```python
from build123d import *

# Parameters (mm, degrees)
F0_R     = 35
F1_DEPTH = 30
F4_DEPTH = 25
F6_D     = 60


with BuildPart() as f1:
    # F0 (on Top) → F1 (new body)
    with BuildSketch(Plane.XY):
        Circle(F0_R)
    extrude(amount=F1_DEPTH)

    # F3 (on offset) → F4 (join)
    with BuildSketch(Plane.YZ.offset(10)):
        Polygon((31.227464, 30), (31.227464, 0), (60.99254, 48.721532), (210.99254, 48.721532), (210.99254, 56.721532), (60.99254, 56.721532), align=None)
    extrude(amount=-F4_DEPTH)

    # F6 (through all)
    with Locations(Plane.XY.offset(30)):
        with Locations((0, 0)):
            Hole(F6_D / 2)


solid = f1.part
```
Verification items for the finished model (mm, model axes). A direction names the side the tool comes from. Give positions to 0.01 mm unless a question says otherwise; leave off trailing zeros. Write each loop counter-clockwise with the first axis right and the second up, starting at its lowest first coordinate (ties: lowest second). Pieces come first, ordered by that corner, then holes. Notation, with made-up numbers: (57, 16.25) - (111, 16.25) arc R30 cw to (111, 52.25) - close; hole circle Ø4 at (-14, 45.5). An arc over 180 degrees is marked (long way). Put each result on its own line as item: value.
Q1. Scan lines: probe 1 along X at (y, z) = (-24, 29); probe 2 along Y at (x, z) = (13.5, 23.5); probe 3 along Y at (x, z) = (-19, 27). Record each from-to range of solid material in increasing order. Write a range as from..to.
Result:
probe 1: -25.48..-18, 18..25.48
probe 2: -32.29..-26.79, 26.79..32.29
probe 3: -29.39..-23.22, 23.22..29.39
Q2. Section check A-A on y = 0. Record the cut outline in (x, z), and give its area (3 significant figures).
Result:
outline: (-35, 0) - (-30, 0) - (-30, 30) - (-35, 30) - close; (30, 0) - (35, 0) - (35, 30) - (30, 30) - close
area: 300 mm2
Q3. Section check B-B on x = -19. Record the cut outline in (y, z).
Result:
outline: (-29.39, 0) - (-23.22, 0) - (-23.22, 30) - (-29.39, 30) - close; (23.22, 0) - (29.39, 0) - (29.39, 30) - (23.22, 30) - close
Q4. Section check C-C on z = 26.5. Record the cut outline in (x, y).
Result:
outline: (-15, 31.62) arc R35 ccw (long way) to (10, 33.54) - (10, 47.42) - (-15, 47.42) - close; hole circle Ø60 at (0, 0)
Q5. Depth check by flat-ended pin: P1, Ø20, axis at x = 1.5, y = 166, coming from the -Z side; P2, Ø1, axis at x = -27, z = 28, coming from the -Y side; P3, Ø8, axis at x = -15, z = 25.5, coming from the -Y side. Enter the tip coordinate at first touch or a pass-through.
Result:
P1: z = 48.72
P2: y = -22.86
P3: y = -33.23
Q6. Set-up check for faces 1 (the face through (-2, 210.993, 53)), 2 (the face through (-2, 135, 48.722)): record each of +Z, -Z, +X, -X, +Y, -Y from which the full face is reachable in a straight line by a thin tool's end or side.
Result:
face 1: +Z, -Z, +X, -X, +Y
face 2: -Z, +X, -X, +Y
Q7. Section check D-D on x = 0.5. Record the cut outline in (y, z).
Result:
outline: (-35, 0) - (-30, 0) - (-30, 30) - (-35, 30) - close; (30, 0) - (35, 0) - (35, 6.17) - (60.99, 48.72) - (210.99, 48.72) - (210.99, 56.72) - (60.99, 56.72) - (31.23, 30) - (30, 30) - close
Q8. Mould release check, pull along Y, two halves, no side actions. Record for faces 3 (the face through (-7.587, -34.168, 14.79)), 4 (the face through (29.97, 1.32, 14.79)), 5 (the face through (-2.32, 46.32, 43.55)), 6 (the face through (-15, 107, 50)): released by +Y, released by -Y, zero draft, split by the parting line, or undercut.
Result:
face 3: split by the parting line
face 4: undercut
face 5: released by -Y
face 6: zero draft
